```python
from build123d import *

# Parameters (mm, degrees)
BOSS_EXTRUDE1_DEPTH      = 2.5
BOSS_EXTRUDE1_DEPTH_BACK = 2.5
SKETCH1_R                = 1.125
SKETCH1_R_2              = 7.05
SKETCH2_W                = 7.5
SKETCH2_H                = 12
BOSS_EXTRUDE2_DEPTH      = 3.5
FILLET3_R                = 2.5
FILLET4_R                = 2.5
FILLET5_R                = 2.5
SKETCH5_R                = 1.5
CUT_EXTRUDE1_DEPTH       = 26.64176281
FILLET3_OF_MIRROR1_R     = 2.5
FILLET4_OF_MIRROR1_R     = 2.5
FILLET5_OF_MIRROR1_R     = 2.5
FILLET6_R                = 2


# Some blends are built 0.0001 mm under size
with BuildPart() as part:
    # Sketch1 → Boss-Extrude1 (new, two sides: drawn at the far end of the back side and taken through both)
    with BuildSketch(Plane(origin=(0, 0, 0), x_dir=(0, 0, -1), z_dir=(1, 0, 0)).offset(-BOSS_EXTRUDE1_DEPTH_BACK)):
        with BuildLine():
            Line((-13, 0), (-13, -3))
            Line((-13, -3), (-13, -14))
            Line((-13, -14), (13, -14))
            Line((13, -14), (13, -3))
            Line((13, -3), (13, 0))
            ThreePointArc((13, 0), (0, 13), (-13, 0))
        make_face()
        with Locations((0, 9)):
            Circle(SKETCH1_R, mode=Mode.SUBTRACT)
        with Locations((9, 0)):
            Circle(SKETCH1_R, mode=Mode.SUBTRACT)
        with Locations((0, -9)):
            Circle(SKETCH1_R, mode=Mode.SUBTRACT)
        with Locations((-9, 0)):
            Circle(SKETCH1_R, mode=Mode.SUBTRACT)
        Circle(SKETCH1_R_2, mode=Mode.SUBTRACT)
    extrude(amount=BOSS_EXTRUDE1_DEPTH + BOSS_EXTRUDE1_DEPTH_BACK)

    # Sketch2 → Boss-Extrude2 (add, symmetric)
    with BuildSketch(Plane(origin=(0, 0, 0), x_dir=(0, 0, -1), z_dir=(1, 0, 0))):
        with Locations((-16.75, -8)):
            Rectangle(SKETCH2_W, SKETCH2_H)
    boss_extrude2 = extrude(amount=BOSS_EXTRUDE2_DEPTH, both=True)

    # Fillet3
    fillet3_edges = [part.edges().sort_by_distance(p)[0] for p in [
        (-3.5, -8, 20.5),
        (3.5, -8, 20.5),
    ]]
    fillet(fillet3_edges, radius=FILLET3_R)

    # Fillet4
    # the kernel refuses this fillet: 2.5 mm, written as the material it takes off along each edge
    with BuildSketch(Plane(origin=(-3.5, 3, 13), x_dir=(0, 0, 1), z_dir=(0, -1, 0))) as fillet4_piece_1:
        with BuildLine():
            CenterArc((2, -2.5), FILLET4_R, 90, 53.130102354)
            Line((0, -1), (-0.04, -0.97))
            ThreePointArc((-0.04, -0.97), (-0.05, -0.5), (-0.05, 0))
            Line((-0.05, 0), (0, 0.05))
            Line((0, 0.05), (2, 0.05))
            Line((2, 0.05), (2, 0))
        make_face()
    extrude(amount=22, mode=Mode.SUBTRACT)
    with BuildSketch(Plane(origin=(3.5, 3, 13), x_dir=(-1, 0, 0), z_dir=(0, -1, 0))) as fillet4_piece_2:
        with BuildLine():
            CenterArc((2.5, -2), FILLET4_R, 126.869897646, 53.130102354)
            Line((0, -2), (-0.05, -2))
            Line((-0.05, -2), (-0.05, 0))
            Line((-0.05, 0), (0, 0.05))
            ThreePointArc((0, 0.05), (0.5, 0.05), (0.97, 0.04))
            Line((0.97, 0.04), (1, 0))
        make_face()
    extrude(amount=22, mode=Mode.SUBTRACT)

    # Fillet5
    fillet5_edges = [part.edges().sort_by_distance(p)[0] for p in [
        (2.5, -8, 13),
        (-2.5, -8, 13),
    ]]
    fillet(fillet5_edges, radius=FILLET5_R)

    # Sketch5 → Cut-Extrude1 (cut, symmetric)
    with BuildSketch(Plane(origin=(0, -2, 0), x_dir=(1, 0, 0), z_dir=(0, 1, 0))):
        with Locations(Location((0, -17.5, 0), (0, 0, 270))):
            Circle(SKETCH5_R)
    cut_extrude1 = extrude(amount=CUT_EXTRUDE1_DEPTH, both=True, mode=Mode.SUBTRACT)

    # Mirror1: Boss-Extrude2, Cut-Extrude1 across plane
    add(boss_extrude2.mirror(Plane.XY))
    add(cut_extrude1.mirror(Plane.XY), mode=Mode.SUBTRACT)

    # Fillet3 of Mirror1
    fillet3_of_mirror1_edges = [part.edges().sort_by_distance(p)[0] for p in [
        (-3.5, -8, -20.5),
        (3.5, -8, -20.5),
    ]]
    fillet(fillet3_of_mirror1_edges, radius=FILLET3_OF_MIRROR1_R)

    # Fillet4 of Mirror1
    # the kernel refuses this fillet: 2.5 mm, written as the material it takes off along each edge
    with BuildSketch(Plane(origin=(-3.5, 3, -13), x_dir=(0, 0, -1), z_dir=(0, -1, 0))) as fillet4_of_mirror1_piece_1:
        with BuildLine():
            CenterArc((2, 2.5), FILLET4_OF_MIRROR1_R, 216.869897646, 53.130102354)
            Line((0, 1), (-0.04, 0.97))
            ThreePointArc((-0.04, 0.97), (-0.05, 0.5), (-0.05, 0))
            Line((-0.05, 0), (0, -0.05))
            Line((0, -0.05), (2, -0.05))
            Line((2, -0.05), (2, 0))
        make_face()
    extrude(amount=22, mode=Mode.SUBTRACT)
    with BuildSketch(Plane(origin=(3.5, 3, -13), x_dir=(0, 0, -1), z_dir=(0, -1, 0))) as fillet4_of_mirror1_piece_2:
        with BuildLine():
            CenterArc((2, -2.5), FILLET4_OF_MIRROR1_R, 90, 53.130102354)
            Line((0, -1), (-0.04, -0.97))
            ThreePointArc((-0.04, -0.97), (-0.05, -0.5), (-0.05, 0))
            Line((-0.05, 0), (0, 0.05))
            Line((0, 0.05), (2, 0.05))
            Line((2, 0.05), (2, 0))
        make_face()
    extrude(amount=22, mode=Mode.SUBTRACT)

    # Fillet5 of Mirror1
    fillet5_of_mirror1_edges = [part.edges().sort_by_distance(p)[0] for p in [
        (2.5, -8, -13),
        (-2.5, -8, -13),
    ]]
    fillet(fillet5_of_mirror1_edges, radius=FILLET5_OF_MIRROR1_R)

    # Fillet6
    fillet6_edges = [part.edges().sort_by_distance(p)[0] for p in [
        (0, -2, 13),
        (0, -2, -13),
    ]]
    fillet(fillet6_edges, radius=FILLET6_R - 0.0001)  # a hair under: the kernel refuses the full size


solid = part.part
```
Check sheet for the modelled part. Datum: model origin and axes. Units: mm. Give positions to 0.01 mm unless a question says otherwise; leave off trailing zeros. Order: outer loops, then holes, each group sorted by start corner. A loop starts at its lowest first (then second) coordinate and runs counter-clockwise, first axis right, second up. Notation, with made-up numbers: M 74.25,82.25 L 112.25,82.25 A11 ccw 112.25,86.25 Z; hole C 10.25,-21.5 d6. An arc over 180 degrees is marked long. Answer in a Markdown table with one row per item. Add a question column.
Q1. Sectioned sample at B-B, the plane z = -17.5. Record the boundary of the cut face in (x, y), and give its area (3 significant figures).
Q2. Release check for a two-part mould opening along Y. For faces 1 (the cylindrical face through (-0.035, 0.338, 7.927)), 2 (the cylindrical face through (-0.04, -1.43, 13.6)), 3 (the flat face through (2.5, -6, 4)) record: released by +Y, released by -Y, zero draft, split by the parting line, or undercut.
Q3. Thickness scan on L1, parallel to Y at x = 0.2, z = 0 (3 decimals); L2, parallel to X at y = -9.75, z = -10; L3, parallel to Z at x = -1.5, y = 2.25. Record the ranges inside material, lowest first.
Q4. Sectioned sample at C-C, the plane y = 4.5. Record the boundary of the cut face in (x, z).
Q5. Gauge pin test, flat ends, axial feed: pin 1 Ø1 at (x, z) = (0, 4) entering from +Y; pin 2 Ø3 at (x, y) = (0, 5) entering from -Z; pin 3 Ø8 at (y, z) = (-1, 5) entering from +X. Record the tip position at first contact, or that the pin passes through.
Q6. Sectioned sample at A-A, the plane x = 0.5. Count the separate pieces of the cut face and the enclosed holes in it, and give its area (3 significant figures).
Q7. Sectioned sample at D-D, the plane z = 0. Record the boundary of the cut face in (x, y) (3 decimals).
Verdict:
| question | item | result |
|---|---|---|
| 1 | outline | M -3.5,-14 L -1.5,-14 L -1.5,-2 L -3.5,-2 Z; M 1.5,-14 L 3.5,-14 L 3.5,-2 L 1.5,-2 Z |
| 1 | area | 48.0 mm² |
| 2 | face 1 | undercut |
| 2 | face 2 | released by +Y |
| 2 | face 3 | zero draft |
| 3 | L1 | -14 to -10.125, -7.875 to -7.05, 7.05 to 7.875, 10.125 to 13 |
| 3 | L2 | -2.5 to 2.5 |
| 3 | L3 | -12.8 to -6.68, 6.68 to 12.8 |
| 4 | outline | M -2.5,-12.2 L 2.5,-12.2 L 2.5,-5.43 L -2.5,-5.43 Z; M -2.5,5.43 L 2.5,5.43 L 2.5,12.2 L -2.5,12.2 Z |
| 5 | pin 1 | y = 12.52 |
| 5 | pin 2 | z = -12.52 |
| 5 | pin 3 | x = 2.5 |
| 6 | separate pieces | 3 |
| 6 | enclosed holes | 5 |
| 6 | area | 571 mm² |
| 7 | outline | M -2.5,-14 L 2.5,-14 L 2.5,-10.125 L -2.5,-10.125 Z; M -2.5,-7.875 L 2.5,-7.875 L 2.5,-7.05 L -2.5,-7.05 Z; M -2.5,7.05 L 2.5,7.05 L 2.5,7.875 L -2.5,7.875 Z; M -2.5,10.125 L 2.5,10.125 L 2.5,13 L -2.5,13 Z |
